from build123d import *

# Parameters (mm, degrees)
F1_DEPTH = 6.35
F3_SIZE  = 3.17499
F4_SIZE  = 3.17499
F2_R     = 11.1125
F5_DEPTH = 25.4
F6_R     = 11.1125
F7_DEPTH = 25.4


# Not quite as in the source:
# - a fillet or chamfer is up to 0.001 mm smaller than in the source, because OpenCascade refuses the exact size


with BuildPart() as f1:
    # F0 (on Top) → F1 (new body)
    with BuildSketch(Plane.XY):
        Polygon((25.4, -15.875), (25.4, 15.875), (16.2345644766, 15.875), (7.0691289532, 0), (16.2345644766, -15.875), align=None)
        Polygon((34.5654355234, 15.875), (25.4, 15.875), (25.4, -15.875), (34.5654355234, -15.875), (43.7308710468, 0), align=None)
        Polygon((7.0691289532, 0), (16.2345644766, 15.875), (-16.2345644766, 15.875), (-7.0691289532, 0), (-16.2345644766, -15.875), (16.2345644766, -15.875), align=None)
        Polygon((-7.0691289532, 0), (-16.2345644766, 15.875), (-25.4, 15.875), (-25.4, -15.875), (-16.2345644766, -15.875), align=None)
        Polygon((-25.4, -15.875), (-25.4, 15.875), (-34.5654355234, 15.875), (-43.7308710468, 0), (-34.5654355234, -15.875), align=None)
    extrude(amount=F1_DEPTH)

    # F3 (size 3.175 in the source; OpenCascade refuses exactly that, so slightly less here)
    f3_edges = [f1.edges().sort_by_distance(p)[0] for p in [
        (-39.148153, -7.9375, 0),
        (-39.148153, 7.9375, 6.35),
        (-39.148153, -7.9375, 6.35),
        (-39.148153, 7.9375, 0),
        (39.148153, -7.9375, 6.35),
        (39.148153, 7.9375, 6.35),
        (39.148153, 7.9375, 0),
        (39.148153, -7.9375, 0),
    ]]
    chamfer(f3_edges, length=F3_SIZE)

    # F4 (size 3.175 in the source; OpenCascade refuses exactly that, so slightly less here)
    f4_edges = [f1.edges().sort_by_distance(p)[0] for p in [
        (0, 15.875, 0),
        (0, 15.875, 6.35),
        (0, -15.875, 6.35),
        (0, -15.875, 0),
    ]]
    chamfer(f4_edges, length=F4_SIZE)

    # F2 (on Top) → F5 (cut)
    with BuildSketch(Plane.XY):
        Circle(F2_R)
    extrude(amount=F5_DEPTH, mode=Mode.SUBTRACT)

    # F6 (on Top) → F7 (cut)
    with BuildSketch(Plane.XY):
        with Locations((26.0964684711, 0)):
            Circle(F6_R)
        with Locations((-26.0964684711, 0)):
            Circle(F6_R)
    extrude(amount=F7_DEPTH, mode=Mode.SUBTRACT)


solid = f1.part
Here's how the part is built. I have some questions about the finished solid (model axes, mm). Coordinates: 2 decimals unless noted, no trailing zeros. Write each loop counter-clockwise with the first axis right and the second up, starting at its lowest first coordinate (ties: lowest second). Pieces come first, ordered by that corner, then holes.
Item 1: I want a section at B-B on z = 5.5. Count the separate pieces of the cut face and the enclosed holes in it, and give its area (3 significant figures).
Item 2: If I drill on line 1 (X direction, y = 6, z = 3); line 2 (X direction, y = 7, z = 1.25); line 3 (Y direction, x = -32, z = 4), over which ranges is the centre line in solid material (lowest first)?
Item 3: I want a section at D-D on z = 1. Write out the boundary of the cut face in (x, y) (1 decimal), and give its area (3 significant figures).
Item 4: Will this pin go through, and if not, where does the flat tip stop? pin 1 (3 mm diameter, centred on y = -4.5, z = 3, fed in from +X).
Item 5: If we mould it in two halves opening along X, with no side actions, what happens to faces 1 (the flat face through (37.818, 7.022, 4.785)), 2 (the flat face through (-37.69, 7.244, 1.565)), 3 (the flat face through (-6.1, 9.5, 6.35)), 4 (the cylindrical face through (14.995, 0.489, 3.131))? For each: +X half, -X half, draft (parallel to the pull), parting line (faces both ways), or undercut.
Findings below:
1. separate pieces: 1
1. enclosed holes: 3
1. area: 849 mm2
2. line 1: x = -40.06 to -35.45, -16.74 to -9.35, 9.35 to 16.74, 35.45 to 40.06
2. line 2: x = -37.47 to -34.73, -17.47 to -8.63, 8.63 to 17.47, 34.73 to 37.47
2. line 3: y = -15.05 to -9.41, 9.41 to 15.05
3. outline: (-41.2, 0) - (-33.3, -13.7) - (33.3, -13.7) - (41.2, 0) - (33.3, 13.7) - (-33.3, 13.7) - close; hole circle Ø22.2 at (-26.1, 0); hole circle Ø22.2 at (0, 0); hole circle Ø22.2 at (26.1, 0)
3. area: 878 mm2
4. pin 1: stops at x = 41.99
5. face 1: +X half
5. face 2: -X half
5. face 3: draft
5. face 4: undercut
